Can you work these out from the model? Positions are in its coordinate system, mm. Face numbers are marked on the shaded views. Round coordinates to 2 decimals unless told otherwise and drop trailing zeros. Loops run counter-clockwise (first coordinate to the right, second up) from the corner with the lowest first, then second, coordinate; pieces in that order, holes last. Notation, with made-up numbers: M 12.5,4 L 40.5,4 A23 ccw 40.5,41 Z; hole C -4.75,77.25 d6. An arc over 180 degrees is marked long. Return JSON: item names as keys, results as strings.
```python
from build123d import *

# Parameters (mm, degrees)
SKETCH1_W           = 38
SKETCH1_H           = 38
SKETCH1_R           = 1
BOSS_EXTRUDE1_DEPTH = 1.3
BOSS_EXTRUDE2_DEPTH = 8.7
SKETCH3_R           = 7
BOSS_EXTRUDE3_DEPTH = 8.6
SKETCH4_R           = 7
BOSS_EXTRUDE4_DEPTH = 30
BOSS_EXTRUDE4_DRAFT = -30


with BuildPart() as part:
    # Sketch1 → Boss-Extrude1 (new body)
    with BuildSketch(Plane(origin=(0, 0, 0), x_dir=(1, 0, 0), z_dir=(0, 1, 0))):
        with Locations((4.613461538, -5.005769231)):
            Rectangle(SKETCH1_W, SKETCH1_H)
        with Locations(Location((-12.386538462, 11.994230769, 0), (0, 0, 270))):
            Circle(SKETCH1_R, mode=Mode.SUBTRACT)
        with Locations(Location((21.613461538, 11.994230769, 0), (0, 0, 270))):
            Circle(SKETCH1_R, mode=Mode.SUBTRACT)
        with Locations(Location((21.613461538, -22.005769231, 0), (0, 0, 270))):
            Circle(SKETCH1_R, mode=Mode.SUBTRACT)
        with Locations(Location((-12.386538462, -22.005769231, 0), (0, 0, 270))):
            Circle(SKETCH1_R, mode=Mode.SUBTRACT)
    extrude(amount=BOSS_EXTRUDE1_DEPTH)

    # Sketch2 → Boss-Extrude2 (add)
    with BuildSketch(Plane(origin=(0, 1.3, 0), x_dir=(1, 0, 0), z_dir=(0, 1, 0))):
        with BuildLine():
            Line((-1.886538462, -11.505769231), (11.113461538, -11.505769231))
            Line((11.113461538, -11.505769231), (11.113461538, -7.333742244))
            Line((11.113461538, -7.333742244), (13.613461538, -7.333742244))
            ThreePointArc((13.613461538, -7.333742244), (15.941434552, -5.005769231), (13.613461538, -2.677796217))
            Line((13.613461538, -2.677796217), (11.113461538, -2.677796217))
            Line((11.113461538, -2.677796217), (11.113461538, 1.494230769))
            Line((11.113461538, 1.494230769), (-1.886538462, 1.494230769))
            Line((-1.886538462, 1.494230769), (-1.886538462, -2.677796217))
            Line((-1.886538462, -2.677796217), (-4.386538462, -2.677796217))
            ThreePointArc((-4.386538462, -2.677796217), (-6.714511475, -5.005769231), (-4.386538462, -7.333742244))
            Line((-4.386538462, -7.333742244), (-1.886538462, -7.333742244))
            Line((-1.886538462, -7.333742244), (-1.886538462, -11.505769231))
        make_face()
    extrude(amount=BOSS_EXTRUDE2_DEPTH)

    # Sketch3 → Boss-Extrude3 (add)
    with BuildSketch(Plane(origin=(0, 10, 0), x_dir=(1, 0, 0), z_dir=(0, 1, 0))):
        with Locations(Location((4.613461538, -5.005769231, 0), (0, 0, 68.213210702))):
            Circle(SKETCH3_R)
    extrude(amount=BOSS_EXTRUDE3_DEPTH)


with BuildPart() as boss_extrude4_tool:
    # Sketch4 → Boss-Extrude4 (with draft: the straight prism first)
    with BuildSketch(Plane(origin=(0, 18.6, 0), x_dir=(1, 0, 0), z_dir=(0, 1, 0))):
        with Locations(Location((4.613461538, -5.005769231, 0), (0, 0, 68.213210702))):
            Circle(SKETCH4_R)
    extrude(amount=BOSS_EXTRUDE4_DEPTH)
    # Boss-Extrude4: the draft: its side faces are tilted about the plane it starts from
    boss_extrude4_sides = [boss_extrude4_tool.faces().sort_by_distance(p)[0] for p in [
        (2.015385327, 33.6, 11.505769231),
    ]]
    draft(boss_extrude4_sides, Plane(origin=(0, 18.6, 0), x_dir=(1, 0, 0), z_dir=(0, 1, 0)), BOSS_EXTRUDE4_DRAFT)


with BuildPart() as part_1:
    add(part.part)

    # Boss-Extrude4: add boss_extrude4_tool
    add(boss_extrude4_tool.part)


solid = part_1.part
```
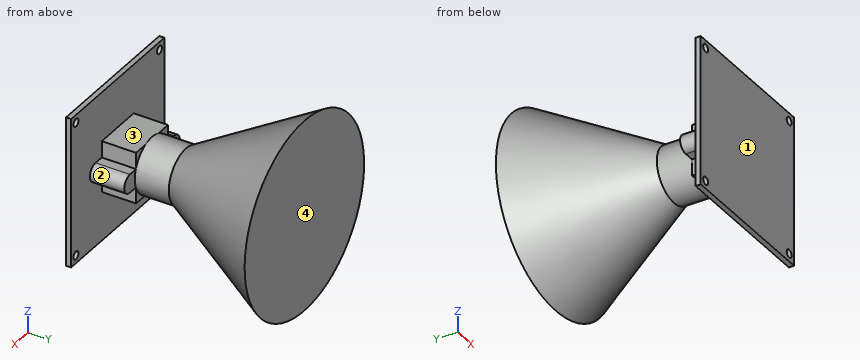
Q1. If I drill on line 1 along Y through (x, z) = (12, 7); line 2 along Y through (x, z) = (-5, 16); line 3 along X through (y, z) = (30.5, 11), over which ranges is the centre line in solid material (lowest first)?
Results:
{"line 1": "y = 0 to 10, 19.73 to 48.6", "line 2": "y = 0 to 1.3, 31.77 to 48.6", "line 3": "x = -7.89 to 17.12"}
Q2. Suppose I cut it at B-B, the plane y = 30.5. Please give me the cut outline in (x, z), plus the area to 3 significant figures.
Results:
{"outline": "C 4.61,5.01 d27.74", "area": "604 mm2"}
Q3. Suppose I cut it at A-A, the plane y = 11. Please give me the cut outline in (x, z).
Results:
{"outline": "C 4.61,5.01 d14"}
Q4. I'm going to push flat-ended pins straight in: pin 1 Ø5 at (x, y) = (21.5, 29.5) entering from -Z; pin 2 Ø1.5 at (y, z) = (35, 2.5) entering from +X; pin 3 Ø3 at (x, y) = (12, 6) entering from -Z; pin 4 Ø1.2 at (x, y) = (-3.5, 4.5) entering from -Z. Where does each tip first touch, or does it pass through?
Results:
{"pin 1": "passes through", "pin 2": "stops at x = 21.34", "pin 3": "stops at z = -1.49", "pin 4": "stops at z = 2.68"}
Q5. Thinking about a two-plate mould opening in Y: for the marked faces 1, 2, 3 and 4, which applies, pulls with the +Y half, pulls with the -Y half, needs draft (parallel to the pull), parting line crosses it, or undercut?
Results:
{"face 1": "pulls with the -Y half", "face 2": "undercut", "face 3": "undercut", "face 4": "pulls with the +Y half"}
